Verification items for the finished model (mm, model axes). Coordinates: 2 decimals unless noted, no trailing zeros. Order: outer loops, then holes, each group sorted by start corner. A loop starts at its lowest first (then second) coordinate and runs counter-clockwise, first axis right, second up. Notation, with made-up numbers: (80.5, 82) -> (84.5, 82) arc R14 cw to (84.5, 90) -> close; hole circle Ø2 at (-8.75, 40). An arc over 180 degrees is marked (long way). Write each question's results on one line, items separated by ' | '. Start each with the question number.
(1) Thickness scan on probe 1 along Y at (x, z) = (30.5, 1.4); probe 2 along Y at (x, z) = (-40.5, 2.3); probe 3 along Y at (x, z) = (-11, 2.95). Record the ranges inside material, lowest first. Write a range as [from, to].
(2) Go/stop test with a flat-tipped pin: pin 1 (3.5 mm diameter, centred on x = 27.82, y = -22.5, fed in from -Z). Record where the tip stops, or that it passes through.
(3) Cross-section at A-A on x = 4.5. Enter the section's corners in (y, z).
(4) Cross-section at D-D on x = -40.5. Enter the section's corners in (y, z), and give its area (3 significant figures).
(5) Cross-section at B-B on y = -22.5. Enter the section's corners in (x, z), and give its area (3 significant figures).
(6) Cross-section at C-C on z = 1.3. Give the number of separate pieces and of enclosed holes in the cut face, and give its area (3 significant figures).
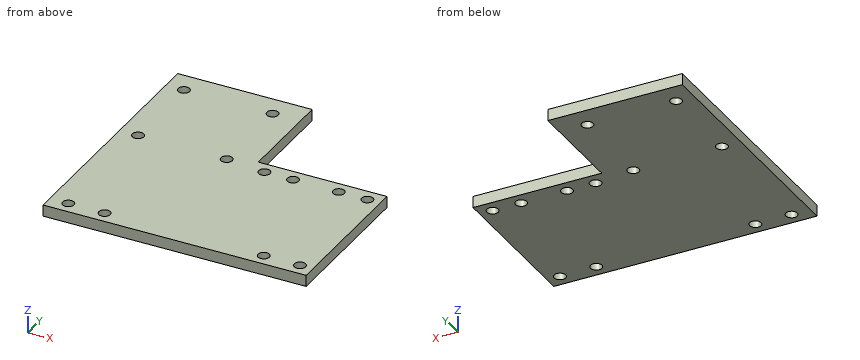
```python
from build123d import *

# Parameters (mm, degrees)
BOSS_EXTRUDE1_DEPTH = 4
SKETCH2_R           = 2
CUT_EXTRUDE1_DEPTH  = 4
SKETCH3_R           = 2
CUT_EXTRUDE2_DEPTH  = 4
SKETCH4_R           = 2
CUT_EXTRUDE3_DEPTH  = 4
SKETCH5_W           = 2
SKETCH5_H           = 90
BOSS_EXTRUDE2_DEPTH = 4
SKETCH6_R           = 2
CUT_EXTRUDE4_DEPTH  = 4


with BuildPart() as part:
    # Sketch1 → Boss-Extrude1 (new body)
    with BuildSketch(Plane.XY):
        Polygon((-45, 27), (-45, 63), (0, 63), (0, 27), (45, 27), (45, -27), (-45, -27), align=None)
    extrude(amount=BOSS_EXTRUDE1_DEPTH)

    # Sketch2 → Cut-Extrude1 (cut)
    with BuildSketch(Plane.XY.offset(4)):
        with Locations((-40.5, -22.5)):
            Circle(SKETCH2_R)
        with Locations((-27.816637329, -22.5)):
            Circle(SKETCH2_R)
        with Locations(Location((27.816637329, -22.5, 0), (0, 0, 180))):
            Circle(SKETCH2_R)
        with Locations(Location((40.5, -22.5, 0), (0, 0, 180))):
            Circle(SKETCH2_R)
        with Locations(Location((30.5, 22.5, 0), (0, 0, 180))):
            Circle(SKETCH2_R)
        with Locations(Location((40.5, 22.5, 0), (0, 0, 180))):
            Circle(SKETCH2_R)
    extrude(amount=-CUT_EXTRUDE1_DEPTH, mode=Mode.SUBTRACT)

    # Sketch3 → Cut-Extrude2 (cut)
    with BuildSketch(Plane.XY.offset(4)):
        with Locations((-40.5, 24.080850084)):
            Circle(SKETCH3_R)
        with Locations((-9.500034607, 24.034529107)):
            Circle(SKETCH3_R)
    extrude(amount=-CUT_EXTRUDE2_DEPTH, mode=Mode.SUBTRACT)

    # Sketch4 → Cut-Extrude3 (cut)
    with BuildSketch(Plane.XY.offset(4)):
        with Locations((-40.690838772, 55.080850084)):
            Circle(SKETCH4_R)
        with Locations((-9.690838772, 55.080850084)):
            Circle(SKETCH4_R)
    extrude(amount=-CUT_EXTRUDE3_DEPTH, mode=Mode.SUBTRACT)

    # Sketch5 → Boss-Extrude2 (add)
    with BuildSketch(Plane.XY.offset(4)):
        with Locations((-46, 18)):
            Rectangle(SKETCH5_W, SKETCH5_H)
    extrude(amount=-BOSS_EXTRUDE2_DEPTH)

    # Sketch6 → Cut-Extrude4 (cut)
    with BuildSketch(Plane.XY.offset(4)):
        with Locations((4.5, 22.5)):
            Circle(SKETCH6_R)
        with Locations((14.5, 22.5)):
            Circle(SKETCH6_R)
    extrude(amount=-CUT_EXTRUDE4_DEPTH, mode=Mode.SUBTRACT)


solid = part.part
```
Results are:
1) probe 1: y = [-27, 20.5], [24.5, 27] | probe 2: y = [-27, -24.5], [-20.5, 22.08], [26.08, 53.09], [57.07, 63] | probe 3: y = [-27, 22.71], [25.36, 53.57], [56.59, 63]
2) pin 1: passes through
3) outline: (-27, 0) -> (20.5, 0) -> (20.5, 4) -> (-27, 4) -> close; (24.5, 0) -> (27, 0) -> (27, 4) -> (24.5, 4) -> close
4) outline: (-27, 0) -> (-24.5, 0) -> (-24.5, 4) -> (-27, 4) -> close; (-20.5, 0) -> (22.08, 0) -> (22.08, 4) -> (-20.5, 4) -> close; (26.08, 0) -> (53.09, 0) -> (53.09, 4) -> (26.08, 4) -> close; (57.07, 0) -> (63, 0) -> (63, 4) -> (57.07, 4) -> close | area: 312 mm2
5) outline: (-47, 0) -> (-42.5, 0) -> (-42.5, 4) -> (-47, 4) -> close; (-38.5, 0) -> (-29.82, 0) -> (-29.82, 4) -> (-38.5, 4) -> close; (-25.82, 0) -> (25.82, 0) -> (25.82, 4) -> (-25.82, 4) -> close; (29.82, 0) -> (38.5, 0) -> (38.5, 4) -> (29.82, 4) -> close; (42.5, 0) -> (45, 0) -> (45, 4) -> (42.5, 4) -> close | area: 304 mm2
6) separate pieces: 1 | enclosed holes: 12 | area: 6,510 mm2
